```python
from build123d import *

# Parameters (mm, degrees)
SKETCH1_W           = 650
SKETCH1_H           = 125
BOSS_EXTRUDE1_DEPTH = 10
SKETCH2_R           = 10
CUT_EXTRUDE2_DEPTH  = 10
SKETCH3_R           = 10
CUT_EXTRUDE3_DEPTH  = 10
BOSS_EXTRUDE3_DEPTH = 20
SKETCH5_W           = 26
SKETCH5_H           = 3
CUT_EXTRUDE4_DEPTH  = 20
BOSS_EXTRUDE4_DEPTH = 20
SKETCH8_R           = 3
CUT_EXTRUDE5_DEPTH  = 20
FILLET1_R           = 50
FILLET2_R           = 40
FILLET3_R           = 50
FILLET4_R           = 40
SKETCH9_R           = 3
CUT_EXTRUDE6_DEPTH  = 10
SKETCH10_W          = 10
SKETCH10_H          = 10
CUT_EXTRUDE7_DEPTH  = 5
CUT_EXTRUDE8_DEPTH  = 30
SKETCH12_W          = 133
SKETCH12_H          = 20
CUT_EXTRUDE9_DEPTH  = 100
SKETCH13_W          = 20
SKETCH13_H          = 36
CUT_EXTRUDE10_DEPTH = 100


with BuildPart() as part:
    # Sketch1 → Boss-Extrude1 (new body)
    with BuildSketch(Plane.XY):
        with Locations((277.89592831, 25.809681948)):
            Rectangle(SKETCH1_W, SKETCH1_H)
    extrude(amount=BOSS_EXTRUDE1_DEPTH)

    # Sketch2 → Cut-Extrude2 (cut)
    with BuildSketch(Plane.XY.offset(10)):
        with Locations((-7.10407169, 48.309681948)):
            Circle(SKETCH2_R)
    extrude(amount=-CUT_EXTRUDE2_DEPTH, mode=Mode.SUBTRACT)

    # Sketch3 → Cut-Extrude3 (cut)
    with BuildSketch(Plane.XY.offset(10)):
        with Locations((562.89592831, 48.309681948)):
            Circle(SKETCH3_R)
    extrude(amount=-CUT_EXTRUDE3_DEPTH, mode=Mode.SUBTRACT)

    # Sketch4 → Boss-Extrude3 (add)
    with BuildSketch(Plane.XY.offset(10)):
        Polygon((32.89592831, 68.309681948), (72.89592831, 68.309681948), (72.89592831, 28.309681948), (32.89592831, 28.309681948), (32.89592831, 35.309681948), (29.89592831, 35.309681948), (29.89592831, 25.309681948), (75.89592831, 25.309681948), (75.89592831, 71.309681948), (29.89592831, 71.309681948), (29.89592831, 61.309681948), (32.89592831, 61.309681948), align=None)
    extrude(amount=BOSS_EXTRUDE3_DEPTH)

    # Sketch5 → Cut-Extrude4 (cut)
    with BuildSketch(Plane.XY.offset(30)):
        with Locations((52.89592831, 69.809681948)):
            Rectangle(SKETCH5_W, SKETCH5_H)
    extrude(amount=-CUT_EXTRUDE4_DEPTH, mode=Mode.SUBTRACT)

    # Sketch7 → Boss-Extrude4 (add)
    with BuildSketch(Plane.XY.offset(10)):
        Polygon((527.89592831, -36.690318052), (463.89592831, -36.690318052), (463.89592831, 25.309681948), (465.89592831, 25.309681948), (465.89592831, -34.690318052), (525.89592831, -34.690318052), (525.89592831, 25.309681948), (527.89592831, 25.309681948), align=None)
        Polygon((458.89592831, 25.309681948), (458.89592831, -36.690318052), (394.89592831, -36.690318052), (394.89592831, 25.309681948), (396.89592831, 25.309681948), (396.89592831, -34.690318052), (456.89592831, -34.690318052), (456.89592831, 25.309681948), align=None)
    extrude(amount=BOSS_EXTRUDE4_DEPTH)

    # Sketch8 → Cut-Extrude5 (cut)
    with BuildSketch(Plane.XY.offset(10)):
        with Locations((177.509070801, 48.309681948)):
            Circle(SKETCH8_R)
        with Locations((377.89592831, 48.309681948)):
            Circle(SKETCH8_R)
    extrude(amount=-CUT_EXTRUDE5_DEPTH, mode=Mode.SUBTRACT)

    # Fillet1
    fillet1_edges = [part.edges().sort_by_distance(p)[0] for p in [
        (602.89592831, -36.690318052, 5),
    ]]
    fillet(fillet1_edges, radius=FILLET1_R)

    # Fillet2
    fillet2_edges = [part.edges().sort_by_distance(p)[0] for p in [
        (602.89592831, 88.309681948, 5),
    ]]
    fillet(fillet2_edges, radius=FILLET2_R)

    # Fillet3
    fillet3_edges = [part.edges().sort_by_distance(p)[0] for p in [
        (-47.10407169, -36.690318052, 5),
    ]]
    fillet(fillet3_edges, radius=FILLET3_R)

    # Fillet4
    fillet4_edges = [part.edges().sort_by_distance(p)[0] for p in [
        (-47.10407169, 88.309681948, 5),
    ]]
    fillet(fillet4_edges, radius=FILLET4_R)

    # Sketch9 → Cut-Extrude6 (cut)
    with BuildSketch(Plane.ZY.offset(47.10407169)):
        with Locations((5, 30.309681948)):
            Circle(SKETCH9_R)
    extrude(amount=-CUT_EXTRUDE6_DEPTH, mode=Mode.SUBTRACT)

    # Sketch10 → Cut-Extrude7 (cut)
    with BuildSketch(Plane.ZY.offset(47.10407169)):
        with Locations((5, 30.309681948)):
            Rectangle(SKETCH10_W, SKETCH10_H)
    extrude(amount=-CUT_EXTRUDE7_DEPTH, mode=Mode.SUBTRACT)

    # Sketch11 → Cut-Extrude8 (cut)
    with BuildSketch(Plane.XY.offset(30)):
        Polygon((29.89592831, 35.309681948), (32.89592831, 35.309681948), (32.89592831, 28.309681948), (72.89592831, 28.309681948), (72.89592831, 35.309681948), (75.89592831, 35.309681948), (75.89592831, 28.309681948), (80.89592831, 28.309681948), (80.89592831, 25.309681948), (75.89592831, 25.309681948), (29.89592831, 25.309681948), (24.89592831, 25.309681948), (24.89592831, 28.309681948), (29.89592831, 28.309681948), align=None)
    extrude(amount=-CUT_EXTRUDE8_DEPTH, mode=Mode.SUBTRACT)

    # Sketch12 → Cut-Extrude9 (cut)
    with BuildSketch(Plane.XZ.offset(36.690318052)):
        with Locations((461.39592831, 20)):
            Rectangle(SKETCH12_W, SKETCH12_H)
    extrude(amount=-CUT_EXTRUDE9_DEPTH, mode=Mode.SUBTRACT)

    # Sketch13 → Cut-Extrude10 (cut)
    with BuildSketch(Plane(origin=(75.89592831, 0, 0), x_dir=(0, 0, -1), z_dir=(1, 0, 0))):
        with Locations((-20, 53.309681948)):
            Rectangle(SKETCH13_W, SKETCH13_H)
    extrude(amount=-CUT_EXTRUDE10_DEPTH, mode=Mode.SUBTRACT)


solid = part.part
```
Verification items for the finished model (mm, model axes). A direction names the side the tool comes from. Coordinates: 2 decimals unless noted, no trailing zeros. Loops run counter-clockwise (first coordinate to the right, second up) from the corner with the lowest first, then second, coordinate; pieces in that order, holes last. Notation, with made-up numbers: (35, -8) - (72, -8) arc R28 ccw to (72, 29) - close; hole circle Ø1 at (48.25, 28.25). An arc over 180 degrees is marked (long way). Answer as a JSON object with one key per item and string values.
(1) Cross-section at B-B, the plane y = 71.5. Record the boundary of the cut face in (x, z).
Response:
{"outline": "(-39.7, 0) - (595.49, 0) - (595.49, 10) - (-39.7, 10) - close"}
(2) Cross-section at A-A, the plane z = 5. Count the separate pieces of the cut face and the enclosed holes in it, then the cut area to 3 significant figures.
Response:
{"separate pieces": "1", "enclosed holes": "5", "area": "78,500 mm²"}
(3) Scan lines: line 1 along X through (y, z) = (30, 8.5); line 2 along X through (y, z) = (26, 1.25); line 3 along X through (y, z) = (54, 8.5). Record each from-to range of solid material in increasing order.
Response:
{"line 1": "x = -42.1 to 29.9, 32.9 to 72.9, 75.9 to 602.9", "line 2": "x = -42.1 to 24.9, 80.9 to 602.9", "line 3": "x = -46.7 to -15.33, 1.12 to 554.67, 571.12 to 602.49"}
(4) Mould release check, pull along Y, two halves, no side actions. Record for faces 4 (the cylindrical face through (587.86, -22.43, 5.07)), 5 (the flat face through (53, 28.31, 5)), 6 (the cylindrical face through (591.49, 76.28, 5.07)), 7 (the flat face through (273, 27, 10)): pulls with the +Y half, pulls with the -Y half, needs draft (parallel to the pull), parting line crosses it, or undercut.
Response:
{"face 4": "pulls with the -Y half", "face 5": "undercut", "face 6": "pulls with the +Y half", "face 7": "needs draft"}
(5) Go/stop test with flat-tipped pins: pin 1 Ø1.5 at (x, z) = (-44, 6) entering from -Y; pin 2 Ø1.5 at (y, z) = (27, 4) entering from -X; pin 3 Ø6 at (x, y) = (215.5, 2) entering from -Z; pin 4 Ø2 at (y, z) = (30.5, 6) entering from -X. Record where each tip stops, or that it passes through.
Response:
{"pin 1": "stops at y = -5.94", "pin 2": "stops at x = -42.1", "pin 3": "stops at z = 0", "pin 4": "stops at x = -37.1"}
(6) Access from +Z, -Z, +X, -X, +Y, -Y to the whole of each face (thin tool, end or side, straight path). Record for faces 1 (the flat face through (-42.104, 33, 3)), 2 (the flat face through (53, 25.31, 5)), 3 (the flat face through (-47.104, 19, 5)).
Response:
{"face 1": "+Z, -Z, -X", "face 2": "+Z, -Z", "face 3": "+Z, -Z, -X, +Y, -Y"}
